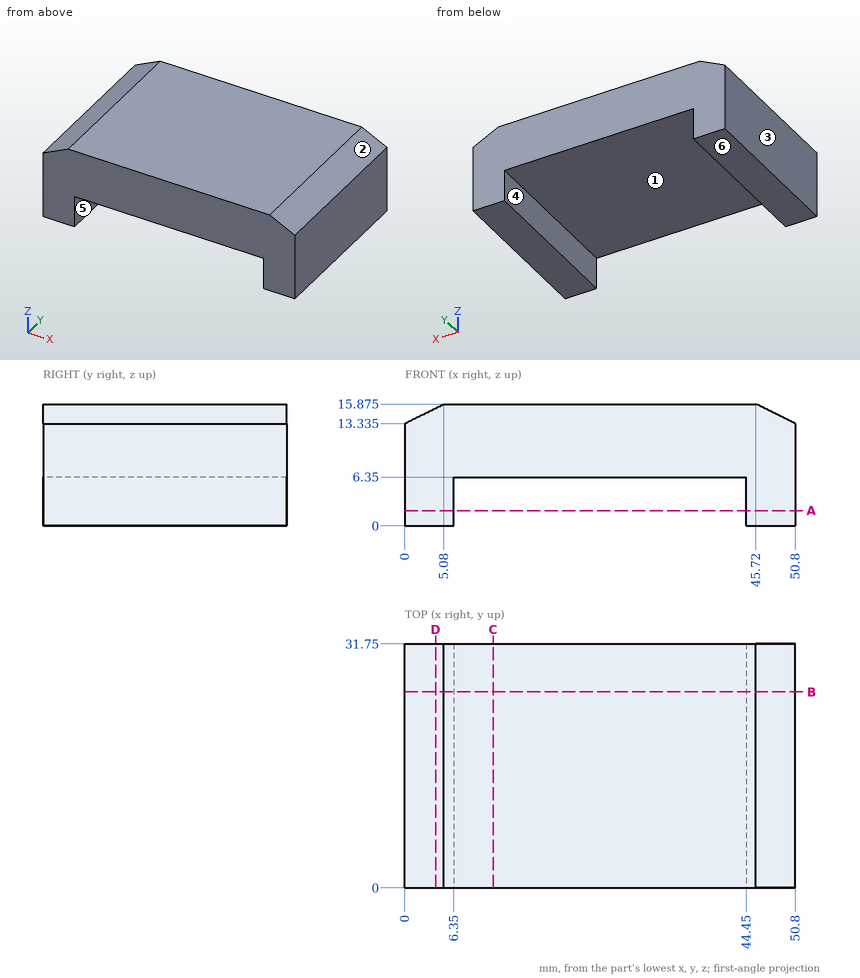
Study the drawing (mm; zero at the part's minimum x, y, z) and answer. A direction names the side the tool comes from. Coordinates: 2 decimals unless noted, no trailing zeros. Loops run counter-clockwise (first coordinate to the right, second up) from the corner with the lowest first, then second, coordinate; pieces in that order, holes last. Notation, with made-up numbers: M 89,32.5 L 139,32.5 A16 cw 139,50.5 Z; hole C -4.75,66.25 d4. An arc over 180 degrees is marked long. Answer as a JSON object with one key per item and string values. Group by question number.
Item 1: Consider L1, parallel to X at y = 28, z = 4.25; L2, parallel to Z at x = 15.5, y = 21 (3 decimals); L3, parallel to X at y = 25.5, z = 14.5. Determine where each line is inside the solid, lowest interval first.
Item 2: Section C-C (x = 11.5) is taken. Write down the section's boundary in (y, z) (3 decimals).
Item 3: Each of these flat-tipped pins is pushed along its axis until it touches: P1, Ø2, axis at x = 26.5, z = 12.5, coming from the -Y side; P2, Ø2, axis at x = 38.5, y = 16, coming from the -Z side. Where does it stop, or does it pass through?
Item 4: Section A-A (z = 2) is taken. Write down the section's boundary in (x, y), and give its area (3 significant figures).
Item 5: Section D-D (x = 4) is taken. Write down the section's boundary in (y, z) (3 decimals), and give its area (3 significant figures).
Item 6: Which of the six approach directions +Z, -Z, +X, -X, +Y, -Y give full straight-line access (tool end or side, diameter ignored) to the marked faces 1 and 2?
Item 7: Section B-B (y = 25.5) is taken. Write down the section's boundary in (x, z) (3 decimals).
Item 8: Determine the mould class of the marked faces 3, 4, 5 and 6 for opening direction X: +X half, -X half, draft (parallel to the pull), parting line (faces both ways), or undercut.
Solved:
{
 "1": {"L1": "x = 0 to 6.35, 44.45 to 50.8", "L2": "z = 6.35 to 15.875", "L3": "x = 2.33 to 48.47"},
 "2": {"outline": "M 0,6.35 L 31.75,6.35 L 31.75,15.875 L 0,15.875 Z"},
 "3": {"P1": "stops at y = 0", "P2": "stops at z = 6.35"},
 "4": {"outline": "M 0,0 L 6.35,0 L 6.35,31.75 L 0,31.75 Z; M 44.45,0 L 50.8,0 L 50.8,31.75 L 44.45,31.75 Z", "area": "403 mm2"},
 "5": {"outline": "M 0,0 L 31.75,0 L 31.75,15.335 L 0,15.335 Z", "area": "487 mm2"},
 "6": {"face 1": "-Z, +Y, -Y", "face 2": "+Z, +X, +Y, -Y"},
 "7": {"outline": "M 0,0 L 6.35,0 L 6.35,6.35 L 44.45,6.35 L 44.45,0 L 50.8,0 L 50.8,13.335 L 45.72,15.875 L 5.08,15.875 L 0,13.335 Z"},
 "8": {"face 3": "-X half", "face 4": "undercut", "face 5": "undercut", "face 6": "draft"}
}
